Design review of the part shown in the three views and the two pictorial views. Dimensions are in mm from the part's minimum x, y and z. A direction names the side the tool comes from. Round coordinates to 2 decimals unless told otherwise and drop trailing zeros. Write each loop counter-clockwise with the first axis right and the second up, starting at its lowest first coordinate (ties: lowest second). Pieces come first, ordered by that corner, then holes. Notation, with made-up numbers: (80.5, -1) - (115.5, -1) arc R8 ccw to (115.5, 7) - close; hole circle Ø1 at (-10.5, -2). An arc over 180 degrees is marked (long way). Use one line per item in the form item = value.
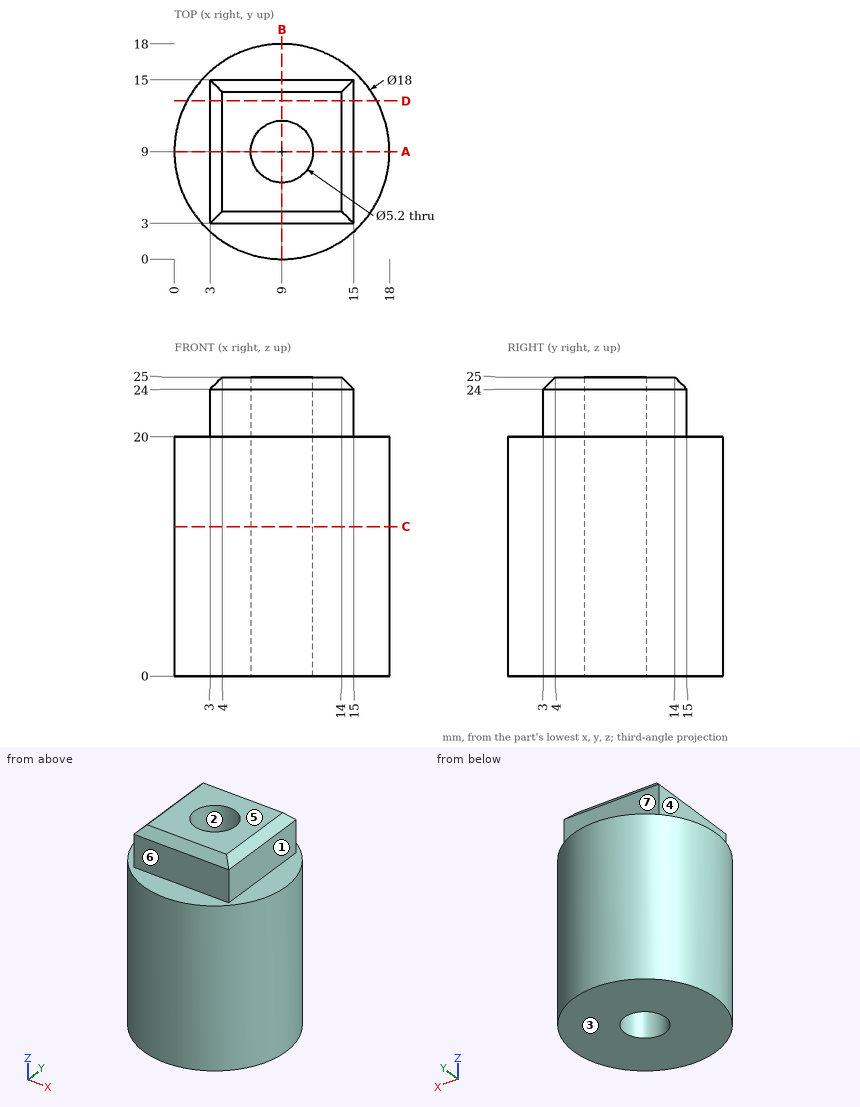
Q1. To check wall thickness, follow line 1 along Y through (x, z) = (9, 15.5); line 2 along X through (y, z) = (10.5, 19); line 3 along X through (y, z) = (14.75, 21). State the ranges of each line that lie inside material, in increasing order. Write a range as from..to.
Calculated:
line_1 = 0..6.4, 11.6..18
line_2 = 0.13..6.88, 11.12..17.87
line_3 = 3..15
Q2. Draft analysis for pull direction X (two halves, no side actions). For the marked faces 1, 2 and 3, state which applies: released by +X, released by -X, zero draft, split by the parting line, or undercut.
Calculated:
face_1 = released by +X
face_2 = undercut
face_3 = zero draft
Q3. We need section C-C on z = 12.5. Write out the cut boundary in (x, y).
Calculated:
outline = circle Ø18 at (9, 9); hole circle Ø5.2 at (9, 9)
Q4. For P1, Ø3, axis at x = 4.5, z = 7, coming from the +Y side; P2, Ø1, axis at x = 13.5, y = 3, coming from the +Z side; P3, Ø3, axis at y = 4, z = 10.5, coming from the +X side, all flat-tipped, find the tip position at first contact; note any pin that passes through.
Calculated:
P1 = 17.49
P2 = 24.5
P3 = 17.29
Q5. Machinability: for the marked faces 4, 5, 6 and 7, which of the approach directions +Z, -Z, +X, -X, +Y, -Y give a long, thin tool a straight path to every point of the face, cutting with its end or side? Answer none if there is none.
Calculated:
face_4 = +Z, -X, +Y, -Y
face_5 = +Z, +X, -X, +Y, -Y
face_6 = +Z, +X, -X, -Y
face_7 = +Z, +X, -X, +Y
Q6. We need section D-D on y = 13.25. Write out the cut boundary in (x, z).
Calculated:
outline = (1.07, 0) - (16.93, 0) - (16.93, 20) - (15, 20) - (15, 24) - (14, 25) - (4, 25) - (3, 24) - (3, 20) - (1.07, 20) - close
Q7. We need section A-A on y = 9. Write out the cut boundary in (x, z), then the cut area to 3 significant figures.
Calculated:
outline = (0, 0) - (6.4, 0) - (6.4, 25) - (4, 25) - (3, 24) - (3, 20) - (0, 20) - close; (11.6, 0) - (18, 0) - (18, 20) - (15, 20) - (15, 24) - (14, 25) - (11.6, 25) - close
area = 289 mm2
